Design review of the part shown in the three views and the two pictorial views. Dimensions are in mm from the part's minimum x, y and z. A direction names the side the tool comes from. Give positions to 0.01 mm unless a question says otherwise; leave off trailing zeros. Loops run counter-clockwise (first coordinate to the right, second up) from the corner with the lowest first, then second, coordinate; pieces in that order, holes last.
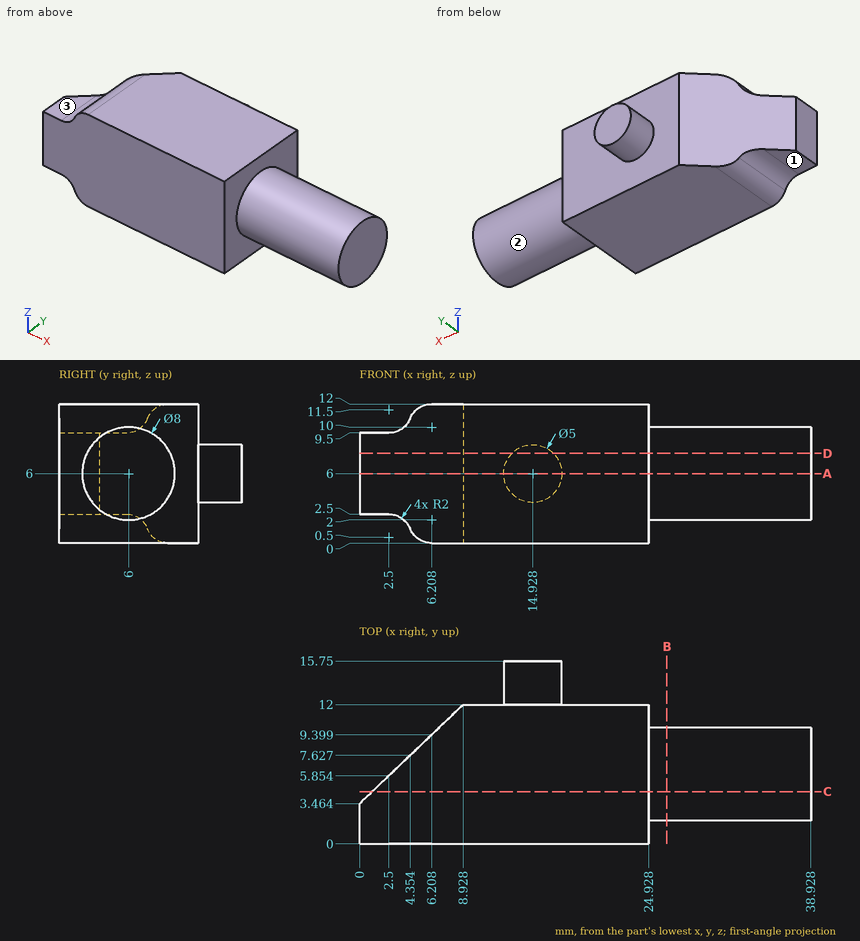
Q1. Consider section A-A on z = 6. Give the boundary of the cut face in (x, y).
Answers:
outline: (0, 0) - (24.93, 0) - (24.93, 2) - (38.93, 2) - (38.93, 10) - (24.93, 10) - (24.93, 12) - (17.43, 12) - (17.43, 15.75) - (12.43, 15.75) - (12.43, 12) - (8.93, 12) - (0, 3.46) - close
Q2. Consider section C-C on y = 4.5. Give the boundary of the cut face in (x, z).
Answers:
outline: (1.08, 2.5) - (2.5, 2.5) arc R2 cw to (4.35, 1.25) arc R2 ccw to (6.21, 0) - (24.93, 0) - (24.93, 2.29) - (38.93, 2.29) - (38.93, 9.71) - (24.93, 9.71) - (24.93, 12) - (6.21, 12) arc R2 ccw to (4.35, 10.75) arc R2 cw to (2.5, 9.5) - (1.08, 9.5) - close
Q3. Consider section B-B on x = 26.5. Give the boundary of the cut face in (y, z).
Answers:
outline: circle Ø8 at (6, 6)
Q4. For probe 1 along X at (y, z) = (1, 8); probe 2 along Y at (x, z) = (12, 3.5); probe 3 along X at (y, z) = (5, 2.25) (1 decimal), list the stretches that pass through material, from the lowest coordinate up.
Answers:
probe 1: x = 0 to 24.93
probe 2: y = 0 to 12
probe 3: x = 3.5 to 38.9
Q5. Consider section D-D on z = 7.75. Give the boundary of the cut face in (x, y), plus the area to 3 significant figures.
Answers:
outline: (0, 0) - (24.93, 0) - (24.93, 2.4) - (38.93, 2.4) - (38.93, 9.6) - (24.93, 9.6) - (24.93, 12) - (16.71, 12) - (16.71, 15.75) - (13.14, 15.75) - (13.14, 12) - (8.93, 12) - (0, 3.46) - close
area: 375 mm2
Q6. For pin 1 Ø5 at (x, z) = (21, 9) entering from +Y; pin 2 Ø1.5 at (y, z) = (5.5, 4) entering from -X (1 decimal); pin 3 Ø0.8 at (x, y) = (1, 4.5) entering from +Z, all flat-tipped, find the tip position at first contact; note any pin that passes through.
Answers:
pin 1: stops at y = 12
pin 2: stops at x = 1.3
pin 3: stops at z = 9.5
Q7. Machinability: for the marked faces 1, 2 and 3, which of the approach directions +Z, -Z, +X, -X, +Y, -Y give a long, thin tool a straight path to every point of the face, cutting with its end or side? Answer none if there is none.
Answers:
face 1: -Z, -X, +Y, -Y
face 2: +X
face 3: +Z, -X, +Y, -Y
